Study the drawing (mm; zero at the part's minimum x, y, z) and answer. A direction names the side the tool comes from. Round coordinates to 2 decimals unless told otherwise and drop trailing zeros. Loops run counter-clockwise (first coordinate to the right, second up) from the corner with the lowest first, then second, coordinate; pieces in that order, holes last. Notation, with made-up numbers: (-10.75, 56.5) - (36.25, 56.5) arc R25 ccw to (36.25, 74.5) - close; hole circle Ø8 at (-6, -31). An arc over 180 degrees is marked (long way). One line per item, written item: value.
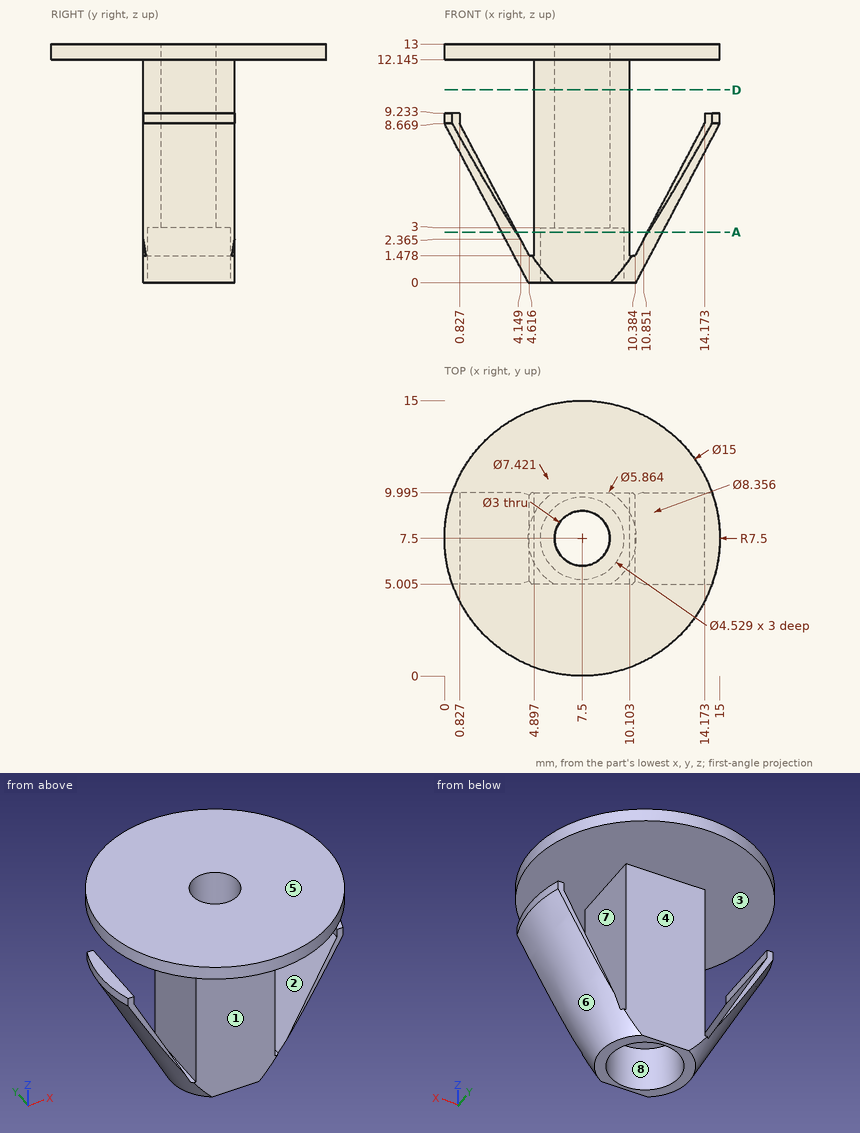
1) Each of these flat-tipped pins is pushed along its axis until it touches: pin 1 Ø1 at (x, y) = (2.5, 11) entering from -Z (1 decimal); pin 2 Ø4 at (x, z) = (12, 7) entering from +Y (1 decimal); pin 3 Ø3 at (x, z) = (13, 5) entering from -Y (1 decimal). Where does it stop, or does it pass through?
Final values:
pin 1: z = 12.1
pin 2: y = 10
pin 3: y = 5
2) A cutting plane is placed at A-A on z = 2.75. Give the number of separate pieces and of enclosed holes in the cut face.
Final values:
separate pieces: 3
enclosed holes: 1
3) For the marked faces 1, 2, 3 and 4, determine the directions among +Z, -Z, +X, -X, +Y, -Y from which every point of the face is accessible in a straight line to the end or side of a thin tool.
Final values:
face 1: -Z, +X, -X, -Y
face 2: +Y, -Y
face 3: none
face 4: -Z, +X, -X, +Y
4) A cutting plane is placed at D-D on z = 10.5. Give the vertices of the cut face in (x, y) (1 decimal).
Final values:
outline: (4.9, 5) - (10.1, 5) - (10.1, 10) - (4.9, 10) - close; hole circle Ø3 at (7.5, 7.5)
5) Consider L1, parallel to Y at x = 7.5, z = 0.9 (1 decimal); L2, parallel to Y at x = 7.5, z = 5.5 (1 decimal); L3, parallel to Y at x = 9.25, z = 12 (1 decimal). Determine where each line is inside the solid, lowest interval first.
Final values:
L1: 5 to 5.2, 9.8 to 10
L2: 5 to 6, 9 to 10
L3: 5 to 10
6) For a pull along X with two mould halves and no side action, classify the marked faces 5, 6, 7 and 8 as released by +X, released by -X, zero draft, split by the parting line, or undercut.
Final values:
face 5: zero draft
face 6: released by +X
face 7: undercut
face 8: undercut
